Autodesk Inventor part; units mm, degrees
ref_plane "YZ Plane" through (0, 0, 0) normal (1, 0, 0) x (0, 1, 0)
ref_plane "XZ Plane" through (0, 0, 0) normal (0, 1, 0) x (-1, 0, 0)
ref_plane "XY Plane" through (0, 0, 0) normal (0, 0, 1) x (1, 0, 0)
sketch "Sketch1" plane through (0, 0, 0) normal (0, 0, 1) x (1, 0, 0)
  circle A0 centre (0, 4.25) radius 4.25
  point P0 (0, 0)
  dimension "d0" = 8.5
  dimension "d1" = 4.25
extrude "Extrusion1" add sketch "Sketch1" along normal mid plane 22.6
sketch "Sketch2" plane through (0, 4.25, 11.3) normal (0, 0, 1) x (1, 0, 0)
  circle A0 centre (0, 0) radius 0.5
  point P0 (0, -4.25)
  dimension "d4" = 1
sketch "Sketch3" plane through (0, 0, 0) normal (1, 0, 0) x (0, 1, 0)
  line L0 (8.5, 11.3) -> (0, 11.3)
  line L1 (4.25, 11.3) -> (4.25, 14)
  line L2 (1.25, 17) -> (-0.9549, 17)
  arc A0 (4.25, 14) -> (1.25, 17) centre (1.25, 14) ccw
  line L3 (-0.9549, 17) -> (-2, 17)
  point P0 (0, 0)
  dimension "d5" = 17
  dimension "d6" = 3
  dimension "d8" = 2
sweep "Sweep1" add profiles "Sketch2" path "Sketch3" path curves L1 A0 L2 L3
mirror "Mirror1" about plane through (0, 0, 0) normal (0, 0, 1) of "Sweep1"
properties part number "MT5-0R05F3_Power_Resistor"
Input: part model. Units: mm. Frame: model coordinates. A direction names the side the tool comes from. Round coordinates to 2 decimals unless told otherwise and drop trailing zeros. Order: outer loops, then holes, each group sorted by start corner. A loop starts at its lowest first (then second) coordinate and runs counter-clockwise, first axis right, second up.
1. Cut plane C-C, the plane x = 3.75. Output: boundary loops of the cut face in (y, z).
The answers:
outline: (2.25, -11.3) - (6.25, -11.3) - (6.25, 11.3) - (2.25, 11.3) - close
2. Mould query, pull axis Z, two halves, no side actions, for faces 4 (the face through (0, -2, 17)), 5 (the face through (-0.065, -0.398, 17.496)). Classes: released by +Z, released by -Z, zero draft, split by the parting line, or undercut.
The answers:
face 4: zero draft
face 5: undercut
3. Cut plane D-D, the plane x = -1.5. Output: boundary loops of the cut face in (y, z), then the cut area to 3 significant figures.
The answers:
outline: (0.27, -11.3) - (8.23, -11.3) - (8.23, 11.3) - (0.27, 11.3) - close
area: 180 mm2
4. Set-up query: faces 1 (the face through (0, -2, -17)), 2 (the face through (-0.065, 3.754, -12.669)), 3 (the face through (-0.065, -0.398, -16.504)). Return all of +Z, -Z, +X, -X, +Y, -Y with unobstructed straight access to the full face (end or side cutting, diameter ignored); none if empty.
The answers:
face 1: +Z, -Z, +X, -X, -Y
face 2: none
face 3: -Y
5. Pin query (flat end, axial travel): P1, Ø2.5, axis at x = 1, y = 2.5, coming from the -Z side; P2, Ø3, axis at x = 2.5, y = 5.5, coming from the -Z side; P3, Ø1, axis at y = 3.5, z = 7.5, coming from the +X side. Return the tip coordinate at first contact, or that it passes through.
The answers:
P1: stops at z = -17.47
P2: stops at z = -11.3
P3: stops at x = 4.24
6. Cut plane B-B, the plane z = -8. Output: boundary loops of the cut face in (x, y), then the cut area to 3 significant figures.
The answers:
outline: circle Ø8.5 at (0, 4.25)
area: 56.7 mm2
7. Material intervals for line 1 (Z direction, x = -2.25, y = 5); line 2 (Y direction, x = 0, z = 12.5); line 3 (X direction, y = 4.5, z = -6), sorted ascending.
The answers:
line 1: z = -11.3 to 11.3
line 2: y = 3.75 to 4.75
line 3: x = -4.24 to 4.24
8. Cut plane A-A, the plane x = 0. Output: boundary loops of the cut face in (y, z).
The answers:
outline: (-2, -17.5) - (1.25, -17.5) arc R3.5 ccw to (4.75, -14) - (4.75, -11.3) - (8.5, -11.3) - (8.5, 11.3) - (4.75, 11.3) - (4.75, 14) arc R3.5 ccw to (1.25, 17.5) - (-2, 17.5) - (-2, 16.5) - (1.25, 16.5) arc R2.5 cw to (3.75, 14) - (3.75, 11.3) - (0, 11.3) - (0, -11.3) - (3.75, -11.3) - (3.75, -14) arc R2.5 cw to (1.25, -16.5) - (-2, -16.5) - close
